from build123d import *

# Parameters (mm, degrees)
SKETCH_1_R               = 2
EXTRUDE_1_DEPTH          = 2
CUT_EXTRUDE_2_DEPTH      = 3
PATTERN_CIRCULAR_1_COUNT = 4


with BuildPart() as part:
    # Эскиз1 → Бобышка-Вытянуть1 (new body)
    with BuildSketch(Plane(origin=(0, 0, 0), x_dir=(1, 0, 0), z_dir=(0, 1, 0))):
        with BuildLine():
            Line((-65, -165.104291208), (65, -165.104291208))
            ThreePointArc((65, -165.104291208), (68.535533906, -163.639825114), (70, -160.104291208))
            Line((70, -160.104291208), (70, -120))
            ThreePointArc((70, -120), (72.928932188, -112.928932188), (80, -110))
            Line((80, -110), (192.768667216, -110))
            ThreePointArc((192.768667216, -110), (196.304201122, -108.535533906), (197.768667216, -105))
            Line((197.768667216, -105), (197.768667216, 105))
            ThreePointArc((197.768667216, 105), (196.304201122, 108.535533906), (192.768667216, 110))
            Line((192.768667216, 110), (80, 110))
            ThreePointArc((80, 110), (72.928932188, 112.928932188), (70, 120))
            Line((70, 120), (70, 160.104291208))
            ThreePointArc((70, 160.104291208), (68.535533906, 163.639825114), (65, 165.104291208))
            Line((65, 165.104291208), (-65, 165.104291208))
            ThreePointArc((-65, 165.104291208), (-68.535533906, 163.639825114), (-70, 160.104291208))
            Line((-70, 160.104291208), (-70, 120))
            ThreePointArc((-70, 120), (-72.928932188, 112.928932188), (-80, 110))
            Line((-80, 110), (-192.768667216, 110))
            ThreePointArc((-192.768667216, 110), (-196.304201122, 108.535533906), (-197.768667216, 105))
            Line((-197.768667216, 105), (-197.768667216, -105))
            ThreePointArc((-197.768667216, -105), (-196.304201122, -108.535533906), (-192.768667216, -110))
            Line((-192.768667216, -110), (-80, -110))
            ThreePointArc((-80, -110), (-72.928932188, -112.928932188), (-70, -120))
            Line((-70, -120), (-70, -160.104291208))
            ThreePointArc((-70, -160.104291208), (-68.535533906, -163.639825114), (-65, -165.104291208))
        make_face()
        with Locations((178.768667216, 0)):
            Circle(SKETCH_1_R, mode=Mode.SUBTRACT)
        with Locations((178.768667216, 80)):
            Circle(SKETCH_1_R, mode=Mode.SUBTRACT)
        with Locations((178.768667216, -80)):
            Circle(SKETCH_1_R, mode=Mode.SUBTRACT)
        with Locations((-178.768667216, -80)):
            Circle(SKETCH_1_R, mode=Mode.SUBTRACT)
        with Locations((-178.768667216, 0)):
            Circle(SKETCH_1_R, mode=Mode.SUBTRACT)
        with Locations((-178.768667216, 80)):
            Circle(SKETCH_1_R, mode=Mode.SUBTRACT)
        with Locations((40, 146.104291208)):
            Circle(SKETCH_1_R, mode=Mode.SUBTRACT)
        with Locations((-40, 146.104291208)):
            Circle(SKETCH_1_R, mode=Mode.SUBTRACT)
        with Locations((-40, -146.104291208)):
            Circle(SKETCH_1_R, mode=Mode.SUBTRACT)
        with Locations((40, -146.104291208)):
            Circle(SKETCH_1_R, mode=Mode.SUBTRACT)
    extrude(amount=EXTRUDE_1_DEPTH)

    # Эскиз5 → Вырез-Вытянуть2 (cut, through all)
    with BuildSketch(Plane.XZ):
        with BuildLine():
            Line((45.596052461, -15), (-45.596052461, -15))
            ThreePointArc((-45.596052461, -15), (-48, 0), (-45.596052461, 15))
            Line((-45.596052461, 15), (45.596052461, 15))
            ThreePointArc((45.596052461, 15), (48, 0), (45.596052461, -15))
        make_face()
    extrude(amount=-CUT_EXTRUDE_2_DEPTH, mode=Mode.SUBTRACT)

    # Эскиз7 → Сверло под метчик  спиральное M51 (revolve, cut)
    with BuildSketch(Plane(origin=(30.0520382, 2, -30.0520382), x_dir=(0, 0, 1), z_dir=(1, 0, 0))):
        Polygon((0, 0), (0, 9.562237609), (2.6, 8), (2.6, 0), align=None)
    hole_wizard_m51 = revolve(axis=Axis((30.0520382, 8.35, -30.0520382), (0, -1, 0)), mode=Mode.SUBTRACT)

    # Круговой массив1: Сверло под метчик  спиральное M51 ×4 about axis
    pattern_circular_1_axis = Axis((0, 0, 0), (0, 1, 0))
    for i in range(1, PATTERN_CIRCULAR_1_COUNT):
        add(hole_wizard_m51.rotate(pattern_circular_1_axis, i * 360 / PATTERN_CIRCULAR_1_COUNT), mode=Mode.SUBTRACT)


solid = part.part
Check sheet for the modelled part. Datum: model origin and axes. Units: mm. Round coordinates to 2 decimals unless told otherwise and drop trailing zeros. Loops run counter-clockwise (first coordinate to the right, second up) from the corner with the lowest first, then second, coordinate; pieces in that order, holes last.
1. Sectioned sample at A-A on z = -139. Record the boundary of the cut face in (x, y).
2. Scan lines: probe 1 along X at (y, z) = (0.5, 80); probe 2 along Z at (x, y) = (-40, 0.5); probe 3 along Z at (x, y) = (3.5, 1.35). Record each from-to range of solid material in increasing order.
3. Gauge pin test, flat ends, axial feed: pin 1 Ø0.6 at (y, z) = (1.5, 146.5) entering from +X; pin 2 Ø0.6 at (y, z) = (0.5, -145) entering from -X. Record the tip position at first contact, or that the pin passes through.
4. Sectioned sample at B-B on x = -103.5. Record the boundary of the cut face in (y, z), and give its area (3 significant figures).
5. Sectioned sample at C-C on y = 0.45. Give the number of separate pieces and of enclosed holes in the cut face, and give its area (3 significant figures).
Recorded:
1. outline: (-70, 0) - (70, 0) - (70, 2) - (-70, 2) - close
2. probe 1: x = -197.77 to -180.77, -176.77 to 176.77, 180.77 to 197.77
2. probe 2: z = -165.1 to -148.1, -144.1 to -15, 15 to 144.1, 148.1 to 165.1
2. probe 3: z = -165.1 to -15, 15 to 165.1
3. pin 1: stops at x = 70
3. pin 2: stops at x = -70
4. outline: (0, -110) - (2, -110) - (2, 110) - (0, 110) - close
4. area: 440 mm2
5. separate pieces: 1
5. enclosed holes: 15
5. area: 99,400 mm2
